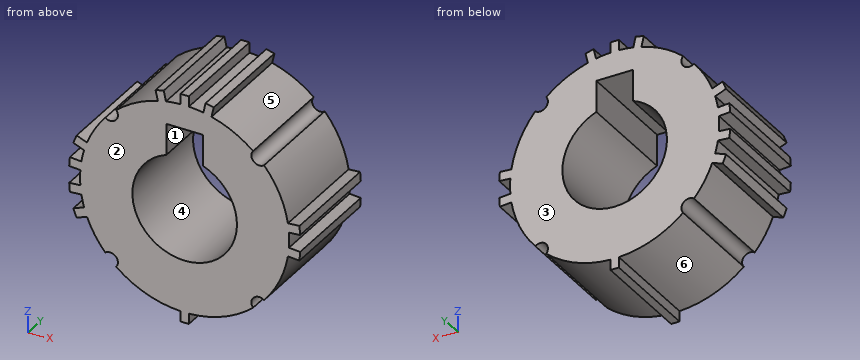
```python
from build123d import *

# Parameters (mm, degrees)
F1_DEPTH = 25.4


with BuildPart() as f1:
    # F0 (on Front) → F1 (new body)
    with BuildSketch(Plane.XZ):
        with BuildLine():
            ThreePointArc((19.284791, 16.530482), (16.762226, 16.687837), (16.616092, 19.211078))
            ThreePointArc((16.616092, 19.211078), (11.870376, 22.455605), (6.516592, 24.549828))
            Line((6.516592, 24.549828), (7.06953, 27.028912))
            Line((7.06953, 27.028912), (5.086263, 27.471263))
            Line((5.086263, 27.471263), (4.533324, 24.992178))
            ThreePointArc((4.533324, 24.992178), (2.781418, 25.247252), (1.016, 25.379672))
            Line((1.016, 25.379672), (1.016, 27.919672))
            Line((1.016, 27.919672), (-1.016, 27.919672))
            Line((-1.016, 27.919672), (-1.016, 25.379672))
            ThreePointArc((-1.016, 25.379672), (-2.781418, 25.247252), (-4.533324, 24.992178))
            Line((-4.533324, 24.992178), (-5.086263, 27.471263))
            Line((-5.086263, 27.471263), (-7.06953, 27.028912))
            Line((-7.06953, 27.028912), (-6.516592, 24.549828))
            ThreePointArc((-6.516592, 24.549828), (-11.870376, 22.455605), (-16.616092, 19.211078))
            ThreePointArc((-16.616092, 19.211078), (-16.762226, 16.687837), (-19.284791, 16.530482))
            ThreePointArc((-19.284791, 16.530482), (-21.815816, 13.00885), (-23.710856, 9.107979))
            Line((-23.710856, 9.107979), (-26.248305, 10.082682))
            Line((-26.248305, 10.082682), (-27.040335, 8.020787))
            Line((-27.040335, 8.020787), (-24.413065, 7.011581))
            ThreePointArc((-24.413065, 7.011581), (-24.787675, 5.543569), (-25.074094, 4.055834))
            Line((-25.074094, 4.055834), (-27.880973, 4.261933))
            Line((-27.880973, 4.261933), (-28.042721, 2.059081))
            Line((-28.042721, 2.059081), (-25.331804, 1.860028))
            ThreePointArc((-25.331804, 1.860028), (-25.4, 0), (-25.331804, -1.860028))
            Line((-25.331804, -1.860028), (-28.042721, -2.059081))
            Line((-28.042721, -2.059081), (-27.880973, -4.261933))
            Line((-27.880973, -4.261933), (-25.074094, -4.055834))
            ThreePointArc((-25.074094, -4.055834), (-24.787675, -5.543569), (-24.413065, -7.011581))
            Line((-24.413065, -7.011581), (-27.040335, -8.020787))
            Line((-27.040335, -8.020787), (-26.248305, -10.082682))
            Line((-26.248305, -10.082682), (-23.710856, -9.107979))
            ThreePointArc((-23.710856, -9.107979), (-21.815816, -13.00885), (-19.284791, -16.530482))
            ThreePointArc((-19.284791, -16.530482), (-16.762226, -16.687837), (-16.616092, -19.211078))
            ThreePointArc((-16.616092, -19.211078), (-9.339997, -23.620424), (-1.016, -25.379672))
            Line((-1.016, -25.379672), (-1.016, -27.919672))
            Line((-1.016, -27.919672), (1.016, -27.919672))
            Line((1.016, -27.919672), (1.016, -25.379672))
            ThreePointArc((1.016, -25.379672), (9.339997, -23.620424), (16.616092, -19.211078))
            ThreePointArc((16.616092, -19.211078), (16.762226, -16.687837), (19.284791, -16.530482))
            ThreePointArc((19.284791, -16.530482), (23.039789, -10.692432), (25.074094, -4.055834))
            Line((25.074094, -4.055834), (27.880973, -4.261933))
            Line((27.880973, -4.261933), (28.042721, -2.059081))
            Line((28.042721, -2.059081), (25.331804, -1.860028))
            ThreePointArc((25.331804, -1.860028), (25.4, 0), (25.331804, 1.860028))
            Line((25.331804, 1.860028), (28.042721, 2.059081))
            Line((28.042721, 2.059081), (27.880973, 4.261933))
            Line((27.880973, 4.261933), (25.074094, 4.055834))
            ThreePointArc((25.074094, 4.055834), (23.039789, 10.692432), (19.284791, 16.530482))
        make_face()
        with BuildLine():
            ThreePointArc((4.445, 11.896721), (0, -12.7), (-4.445, 11.896721))
            Line((-4.445, 11.896721), (-4.445, 19.516721))
            Line((-4.445, 19.516721), (4.445, 19.516721))
            Line((4.445, 19.516721), (4.445, 11.896721))
        make_face(mode=Mode.SUBTRACT)
    extrude(amount=F1_DEPTH)


solid = f1.part
```
Geometry: final body of the model. Coordinates: model frame, mm. Face numbers are marked on the shaded views. A direction names the side the tool comes from. Give positions to 0.01 mm unless a question says otherwise; leave off trailing zeros. Loops run counter-clockwise (first coordinate to the right, second up) from the corner with the lowest first, then second, coordinate; pieces in that order, holes last. Notation, with made-up numbers: (17.25, 5) -> (74.25, 5) arc R20 cw to (74.25, 42) -> close; hole circle Ø11 at (45.5, 3.5). An arc over 180 degrees is marked (long way). Use CSV: the item, a comma, the result in double quotes.
(1) Cut plane B-B (x = 0). Output: boundary loops of the cut face in (y, z).
From the geometry:
outline,"(-25.4, -27.92) -> (0, -27.92) -> (0, -12.7) -> (-25.4, -12.7) -> close; (-25.4, 19.52) -> (0, 19.52) -> (0, 27.92) -> (-25.4, 27.92) -> close"
(2) Cut plane D-D (z = -21). Output: boundary loops of the cut face in (x, y), plus the area to 3 significant figures.
From the geometry:
outline,"(-14.29, -25.4) -> (14.29, -25.4) -> (14.29, 0) -> (-14.29, 0) -> close"
area,"726 mm^2"
(3) Pull-direction query (X, two-part tool) for the marked faces 3, 4, 5 and 6; classes: released by +X, released by -X, zero draft, split by the parting line, or undercut.
From the geometry:
face 3,"zero draft"
face 4,"undercut"
face 5,"released by +X"
face 6,"released by -X"
(4) Cut plane A-A (z = 0). Output: boundary loops of the cut face in (x, y).
From the geometry:
outline,"(-25.4, -25.4) -> (-12.7, -25.4) -> (-12.7, 0) -> (-25.4, 0) -> close; (12.7, -25.4) -> (25.4, -25.4) -> (25.4, 0) -> (12.7, 0) -> close"
(5) First-contact query: P1, Ø2, axis at y = -12.5, z = -26.5, coming from the -X side; P2, Ø2, axis at x = -9.5, z = -3, coming from the -Y side (1 decimal); P3, Ø3, axis at y = -22, z = -4.5, coming from the -X side; P4, Ø1.5, axis at x = 18.5, y = -3, coming from the +Z side. Flat tips, straight axial feed; report the tip coordinate or a pass-through.
From the geometry:
P1,"x = -1.02"
P2,"through"
P3,"x = -27.97"
P4,"z = 16.5"
(6) Ray query, line 1 along X through (y, z) = (-9.75, 0); line 2 along Z through (x, y) = (-0.5, -8); line 3 along X through (y, z) = (-5, -11.5). Return the intervals inside material, ascending. Write a range as [from, to].
From the geometry:
line 1,"[-25.4, -12.7], [12.7, 25.4]"
line 2,"[-27.92, -12.69], [19.52, 27.92]"
line 3,"[-22.65, -5.39], [5.39, 22.65]"
(7) Access query for the marked faces 1 and 2. Directions: +Z, -Z, +X, -X, +Y, -Y. A direction counts if a zero-diameter tool reaches every point of the face in a straight line with its end or side. Return the directions, or none.
From the geometry:
face 1,"+Y, -Y"
face 2,"+Z, -Z, +X, -X, -Y"
(8) Cut plane C-C (x = -14). Output: boundary loops of the cut face in (y, z).
From the geometry:
outline,"(-25.4, -21.19) -> (0, -21.19) -> (0, 21.19) -> (-25.4, 21.19) -> close"
